from build123d import *

# Parameters (mm, degrees)
F0_W     = 109.156876
F0_H     = 67.89817
F0_W_2   = 94.212786
F0_H_2   = 54.903298
F1_DEPTH = 54.61
F2_W     = 45.806905
F2_H     = 23.568978
F3_DEPTH = 67.899169
F4_R     = 6.891568
F5_DEPTH = 109.157877


with BuildPart() as f1:
    # F0 (on Top) → F1 (new body)
    with BuildSketch(Plane.XY):
        Rectangle(F0_W, F0_H)
        Rectangle(F0_W_2, F0_H_2, mode=Mode.SUBTRACT)
    extrude(amount=F1_DEPTH)

    # F2 (on face) → F3 (cut, through all)
    with BuildSketch(Plane.XZ.offset(33.949085)):
        with Locations((0.162437, 42.825511)):
            Rectangle(F2_W, F2_H)
    extrude(amount=-F3_DEPTH, mode=Mode.SUBTRACT)

    # F4 (on face) → F5 (cut, through all)
    with BuildSketch(Plane.YZ.offset(54.578438)):
        with Locations((0, 41.11205)):
            Circle(F4_R)
    extrude(amount=-F5_DEPTH, mode=Mode.SUBTRACT)


solid = f1.part
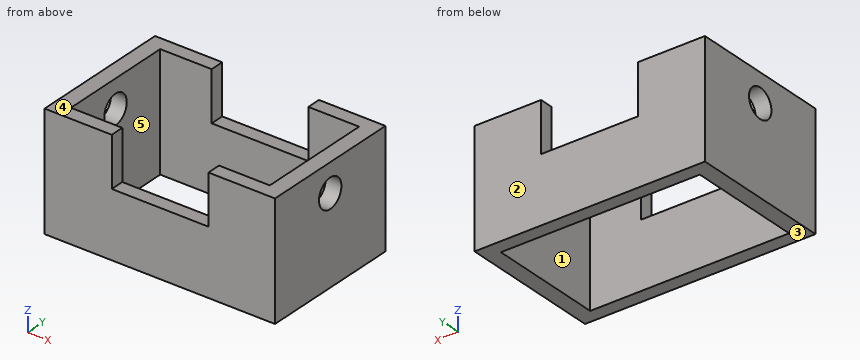
Design review of the part built by this model. Coordinates are the model's own, in mm. Face numbers are marked on the shaded views. A direction names the side the tool comes from. Round coordinates to 2 decimals unless told otherwise and drop trailing zeros. Order: outer loops, then holes, each group sorted by start corner. A loop starts at its lowest first (then second) coordinate and runs counter-clockwise, first axis right, second up.
1) For L1, parallel to X at y = 5, z = 26.5; L2, parallel to Z at x = -51, y = 0; L3, parallel to Y at x = 20, z = 27, list the stretches that pass through material, from the lowest coordinate up.
The answers:
L1: x = -54.58 to -47.11, 47.11 to 54.58
L2: z = 0 to 34.22, 48 to 54.61
L3: y = -33.95 to -27.45, 27.45 to 33.95
2) Consider section D-D (z = 19.5). State the section outline as (x, y) points, plus the area to 3 significant figures.
The answers:
outline: (-54.58, -33.95) - (54.58, -33.95) - (54.58, 33.95) - (-54.58, 33.95) - close; hole (-47.11, -27.45) - (47.11, -27.45) - (47.11, 27.45) - (-47.11, 27.45) - close
area: 2,240 mm2
3) Consider section A-A (y = 0). State the section outline as (x, z) points, plus the area to 3 significant figures.
The answers:
outline: (-54.58, 0) - (-47.11, 0) - (-47.11, 34.22) - (-54.58, 34.22) - close; (-54.58, 48) - (-47.11, 48) - (-47.11, 54.61) - (-54.58, 54.61) - close; (47.11, 0) - (54.58, 0) - (54.58, 34.22) - (47.11, 34.22) - close; (47.11, 48) - (54.58, 48) - (54.58, 54.61) - (47.11, 54.61) - close
area: 610 mm2
4) Consider section B-B (x = 44). State the section outline as (y, z) points.
The answers:
outline: (-33.95, 0) - (-27.45, 0) - (-27.45, 54.61) - (-33.95, 54.61) - close; (27.45, 0) - (33.95, 0) - (33.95, 54.61) - (27.45, 54.61) - close
5) Clearance check with a flat-ended pin moving along its axis: pin 1 Ø3 at (x, y) = (-10.5, 29.5) entering from +Z. State where the tip first meets the part, or that it passes through.
The answers:
pin 1: stops at z = 31.04
6) Consider section C-C (y = -8.5). State the section outline as (x, z) points, plus the area to 3 significant figures.
The answers:
outline: (-54.58, 0) - (-47.11, 0) - (-47.11, 54.61) - (-54.58, 54.61) - close; (47.11, 0) - (54.58, 0) - (54.58, 54.61) - (47.11, 54.61) - close
area: 816 mm2
7) Machinability: for the marked faces 4 and 5, which of the approach directions +Z, -Z, +X, -X, +Y, -Y give a long, thin tool a straight path to every point of the face, cutting with its end or side? Answer none if there is none.
The answers:
face 4: +Z, +X, -X, +Y, -Y
face 5: +Z, -Z
8) Draft analysis for pull direction Y (two halves, no side actions). For the marked faces 1, 2 and 3, state which applies: released by +Y, released by -Y, zero draft, split by the parting line, or undercut.
The answers:
face 1: undercut
face 2: released by +Y
face 3: zero draft
